Work out the finished part from the listing and answer in its coordinate system (mm). A direction names the side the tool comes from. Round coordinates to 2 decimals unless told otherwise and drop trailing zeros. Write each loop counter-clockwise with the first axis right and the second up, starting at its lowest first coordinate (ties: lowest second). Pieces come first, ordered by that corner, then holes. Notation, with made-up numbers: M 3.25,20.5 L 14.25,20.5 A13 cw 14.25,33.5 Z; hole C 33,61 d2. An arc over 180 degrees is marked long. One line per item, written item: value. Start each with the question number.
Q1. Find section A-A (x = -2). Write down the section's boundary in (y, z), and give its area (3 significant figures).
Q2. Consider probe 1 along X at (y, z) = (0.5, 20); probe 2 along Z at (x, y) = (9.5, 1.5); probe 3 along Z at (x, y) = (-12, 0.25). Determine where each line is inside the solid, lowest interval first.
Q3. Given pin 1 Ø5 at (x, y) = (13.5, 1.5) entering from -Z; pin 2 Ø4 at (y, z) = (-0.5, 21.5) entering from -X; pin 3 Ø5 at (x, y) = (-9.5, 2.5) entering from +Z; pin 4 Ø2.5 at (x, y) = (-13.8, 0) entering from +Z, each flat-ended and moving along its own axis, determine where each tip first touches the part or whether it passes through.
Q4. Find section B-B (y = 4.25). Write down the section's boundary in (x, z).
Q5. A tool of negligible diameter and unlimited length cuts with its end or side. For faces 4 (the cylindrical face through (-9.36, -3.9, 0.49)), 5 (the flat face through (-11.5, 0, 20)), 6 (the flat face through (11.5, 0, 8)), from which of +Z, -Z, +X, -X, +Y, -Y can it reach the whole face along a straight path? Write none if from no direction.
Q6. The mould has two halves that part along X. Classify faces 1 (the flat face through (16, -3, 17)), 2 (the flat face through (-2, 0, 27)), 3 (the cylindrical face through (-12.3, -0.1, 17)): released by +X, released by -X, zero draft, split by the parting line, or undercut.
Q7. Find section C-C (z = 28). Write down the section's boundary in (x, y).
from build123d import *

# Parameters (mm, degrees)
SKETCH_1_W               = 23
SKETCH_1_H               = 12
EXTRUDE_1_DEPTH          = 16
SKETCH_2_W               = 32
SKETCH_2_H               = 12
EXTRUDE_2_DEPTH          = 2
SKETCH_3_W               = 23
SKETCH_3_H               = 12
EXTRUDE_3_DEPTH          = 5
EXTRUDE_4_DEPTH          = 4
SKETCH_6_R               = 2
EXTRUDE_5_DEPTH          = 4
CUT_EXTRUDE_1_DEPTH      = 4
SKETCH_9_R               = 3
CUT_EXTRUDE_2_DEPTH      = 1
MIRROR_3_COPY_1_SKETCH_R = 3
MIRROR_3_COPY_1_DEPTH    = 1


with BuildPart() as part:
    # 草图1 → 凸台-拉伸1 (new body)
    with BuildSketch(Plane.XY):
        Rectangle(SKETCH_1_W, SKETCH_1_H)
    extrude(amount=EXTRUDE_1_DEPTH)

    # 草图2 → 凸台-拉伸2 (add)
    with BuildSketch(Plane.XY.offset(16)):
        Rectangle(SKETCH_2_W, SKETCH_2_H)
    extrude(amount=EXTRUDE_2_DEPTH)

    # 草图3 → 凸台-拉伸3 (add)
    with BuildSketch(Plane.XY.offset(18)):
        Rectangle(SKETCH_3_W, SKETCH_3_H)
    extrude(amount=EXTRUDE_3_DEPTH)

    # 草图4 → 凸台-拉伸4 (add)
    with BuildSketch(Plane.XY.offset(23)):
        with BuildLine():
            Line((1.631262932, 2), (0.156854249, 2))
            ThreePointArc((0.156854249, 2), (-11.5, 0), (0.156854249, -2))
            Line((0.156854249, -2), (1.631262932, -2))
            ThreePointArc((1.631262932, -2), (3.631262932, 0), (1.631262932, 2))
        make_face()
    extrude(amount=EXTRUDE_4_DEPTH)

    # 草图6 → 凸台-拉伸5 (add)
    with BuildSketch(Plane.XY.offset(27)):
        with Locations((-5.5, 0)):
            Circle(SKETCH_6_R)
    extrude(amount=EXTRUDE_5_DEPTH)

    # 草图8 → 切除-拉伸1 (cut)
    with BuildSketch(Plane.XY.offset(18)):
        with BuildLine():
            Line((15.211851697, 0.5), (16, 0.5))
            Line((16, 0.5), (16, -0.5))
            Line((16, -0.5), (15.211851697, -0.5))
            ThreePointArc((15.211851697, -0.5), (12.297638134, 0), (15.211851697, 0.5))
        make_face()
    cut_extrude_1 = extrude(amount=-CUT_EXTRUDE_1_DEPTH, mode=Mode.SUBTRACT)

    # 镜向1: 切除-拉伸1 across plane
    add(cut_extrude_1.mirror(Plane(origin=(0, 0, 0), x_dir=(0, 0, 1), z_dir=(1, 0, 0))), mode=Mode.SUBTRACT)

    # 草图9 → 切除-拉伸2 (cut)
    with BuildSketch(Plane(origin=(0, 0, 0), x_dir=(-1, 0, 0), z_dir=(0, 0, -1))):
        with Locations((11.5, 6)):
            Circle(SKETCH_9_R)
    cut_extrude_2 = extrude(amount=-CUT_EXTRUDE_2_DEPTH, mode=Mode.SUBTRACT)

    # 镜向2: 切除-拉伸2 across plane
    add(cut_extrude_2.mirror(Plane(origin=(0, 0, 0), x_dir=(0, 0, 1), z_dir=(1, 0, 0))), mode=Mode.SUBTRACT)

    # 镜向3: 切除-拉伸2 across plane
    add(cut_extrude_2.mirror(Plane.ZX), mode=Mode.SUBTRACT)

    # 镜向3 copy 1 sketch → 镜向3 copy 1 (cut)
    with BuildSketch(Plane(origin=(0, 0, 0), x_dir=(1, 0, 0), z_dir=(0, 0, -1))):
        with Locations((11.5, 6)):
            Circle(MIRROR_3_COPY_1_SKETCH_R)
    extrude(amount=-MIRROR_3_COPY_1_DEPTH, mode=Mode.SUBTRACT)


solid = part.part
The answers:
1. outline: M -6,0 L 6,0 L 6,23 L 4.87,23 L 4.87,27 L -4.87,27 L -4.87,23 L -6,23 Z
1. area: 315 mm2
2. probe 1: -11.5 to 11.5
2. probe 2: 0 to 23
2. probe 3: 16 to 18
3. pin 1: z = 0
3. pin 2: x = -11.5
3. pin 3: z = 27
3. pin 4: through
4. outline: M -16,16 L -11.5,16 L -11.5,1 L -9.06,1 L -9.06,0 L 9.06,0 L 9.06,1 L 11.5,1 L 11.5,16 L 16,16 L 16,18 L 11.5,18 L 11.5,23 L -1.26,23 L -1.26,27 L -9.74,27 L -9.74,23 L -11.5,23 L -11.5,18 L -16,18 Z
5. face 4: -Z, -X, -Y
5. face 5: +Z, -X, +Y, -Y
5. face 6: -Z, +X, +Y, -Y
6. face 1: released by +X
6. face 2: zero draft
6. face 3: undercut
7. outline: C -5.5,0 d4
